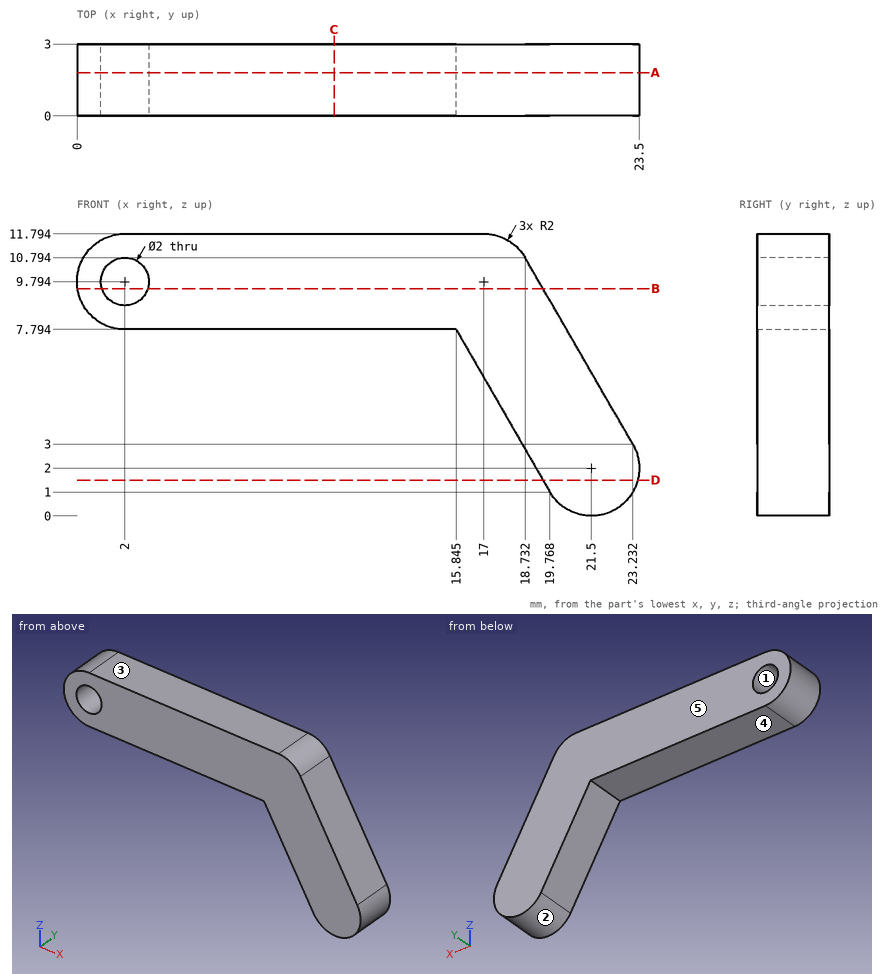
Geometry: see drawing. Coordinates: mm, zero at the bounding-box minimum. A direction names the side the tool comes from. Give positions to 0.01 mm unless a question says otherwise; leave off trailing zeros. Write each loop counter-clockwise with the first axis right and the second up, starting at its lowest first coordinate (ties: lowest second). Pieces come first, ordered by that corner, then holes. Notation, with made-up numbers: M 67.5,87 L 113.5,87 A22 ccw 113.5,107 Z; hole C 89,57 d11. An arc over 180 degrees is marked long. Answer in a Markdown table with one row per item. Add a question column.
(1) Ray query, line 1 (Z direction, x = 2, y = 1.75); line 2 (Z direction, x = 3.25, y = 0.4); line 3 (X direction, y = 2.7, z = 9.25) (1 decimal). Return the intervals inside material, ascending.
(2) Mould query, pull axis Z, two halves, no side actions, for the marked faces 1, 2 and 3. Classes: +Z half, -Z half, draft (parallel to the pull), parting line (faces both ways), or undercut.
(3) Section A-A on y = 1.8. Return loops of the section in (x, z) (1 decimal).
(4) First-contact query: pin 1 (1.5 mm diameter, centred on y = 2, z = 5, fed in from -X) (1 decimal); pin 2 (1 mm diameter, centred on y = 0.5, z = 7, fed in from +X). Flat tips, straight axial feed; report the tip coordinate or a pass-through.
(5) Section D-D on z = 1.5. Return loops of the section in (x, y).
(6) Section C-C on x = 10.75. Return loops of the section in (y, z), and give its area (3 significant figures).
(7) Section B-B on z = 9.5. Return loops of the section in (x, y).
(8) Reachability of the marked faces 4 and 5 from +Z, -Z, +X, -X, +Y, -Y: full face, straight path, thin tool, end or side. Return the list, or none.
Result set:
| question | item | result |
|---|---|---|
| 1 | line 1 | z = 7.79 to 8.79, 10.79 to 11.79 |
| 1 | line 2 | z = 7.79 to 11.79 |
| 1 | line 3 | x = 0.1 to 1.2, 2.8 to 19.6 |
| 2 | face 1 | undercut |
| 2 | face 2 | parting line |
| 2 | face 3 | +Z half |
| 3 | outline | M 2,7.8 L 15.8,7.8 L 19.8,1 A2 ccw 23.2,3 L 18.7,10.8 A2 ccw 17,11.8 L 2,11.8 A2 ccw Z; hole C 2,9.8 d2 |
| 4 | pin 1 | stops at x = 17 |
| 4 | pin 2 | stops at x = 21.21 |
| 5 | outline | M 19.48,0 L 23.44,0 L 23.44,3 L 19.48,3 Z |
| 6 | outline | M 0,7.79 L 3,7.79 L 3,11.79 L 0,11.79 Z |
| 6 | area | 12.0 mm^2 |
| 7 | outline | M 0.02,0 L 1.04,0 L 1.04,3 L 0.02,3 Z; M 2.96,0 L 19.48,0 L 19.48,3 L 2.96,3 Z |
| 8 | face 4 | -Z, -X, +Y, -Y |
| 8 | face 5 | +Z, -Z, +X, -X, +Y |
